from build123d import *

# Parameters (mm, degrees)
SKETCH1_W       = 22
SKETCH1_H       = 22
EXTRUDE1_DEPTH  = 7
SKETCH2_W       = 7
SKETCH2_H       = 7
EXTRUDE2_DEPTH  = 7
SKETCH3_W       = 7
SKETCH3_H       = 4
SKETCH3_W_2     = 4
SKETCH3_H_2     = 7
EXTRUDE3_DEPTH  = 7
SKETCH4_W       = 4
SKETCH4_H       = 4
EXTRUDE5_DEPTH  = 7
SKETCH5_R       = 2.55
EXTRUDE6_DEPTH  = 10
SKETCH6_R       = 1.025
EXTRUDE7_DEPTH  = 10
SKETCH7_R       = 1.025
EXTRUDE8_DEPTH  = 10
SKETCH8_R       = 1.025
EXTRUDE9_DEPTH  = 10
SKETCH9_R       = 1.025
EXTRUDE10_DEPTH = 10


with BuildPart() as part:
    # Sketch1 → Extrude1 (new body)
    with BuildSketch(Plane.XY):
        Rectangle(SKETCH1_W, SKETCH1_H)
    extrude(amount=EXTRUDE1_DEPTH)

    # Sketch2 → Extrude2 (cut)
    with BuildSketch(Plane.XY.offset(7)):
        with Locations((7.5, 7.5)):
            Rectangle(SKETCH2_W, SKETCH2_H)
        with Locations((-7.5, 7.5)):
            Rectangle(SKETCH2_W, SKETCH2_H)
        with Locations((-7.5, -7.5)):
            Rectangle(SKETCH2_W, SKETCH2_H)
        with Locations((7.5, -7.5)):
            Rectangle(SKETCH2_W, SKETCH2_H)
    extrude(amount=-EXTRUDE2_DEPTH, mode=Mode.SUBTRACT)

    # Sketch3 → Extrude3 (cut)
    with BuildSketch(Plane.XY.offset(7)):
        with Locations((-7.5, 0)):
            Rectangle(SKETCH3_W, SKETCH3_H)
        with Locations((0, 7.5)):
            Rectangle(SKETCH3_W_2, SKETCH3_H_2)
        with Locations((7.5, 0)):
            Rectangle(SKETCH3_W, SKETCH3_H)
        with Locations((0, -7.5)):
            Rectangle(SKETCH3_W_2, SKETCH3_H_2)
        Rectangle(SKETCH3_W_2, SKETCH3_H)
    extrude(amount=-EXTRUDE3_DEPTH, mode=Mode.SUBTRACT)

    # Sketch4 → Extrude5 (add)
    with BuildSketch(Plane.XY.offset(7)):
        Rectangle(SKETCH4_W, SKETCH4_H)
    extrude(amount=-EXTRUDE5_DEPTH)

    # Sketch5 → Extrude6 (cut)
    with BuildSketch(Plane.XY.offset(7)):
        Circle(SKETCH5_R)
    extrude(amount=-EXTRUDE6_DEPTH, mode=Mode.SUBTRACT)

    # Sketch6 → Extrude7 (cut)
    with BuildSketch(Plane(origin=(4, 0, 0), x_dir=(0, 0, -1), z_dir=(1, 0, 0))):
        with Locations((-3.14721043, 9.031360998)):
            Circle(SKETCH6_R)
    extrude(amount=-EXTRUDE7_DEPTH, mode=Mode.SUBTRACT)

    # Sketch7 → Extrude8 (cut)
    with BuildSketch(Plane.XZ.offset(4)):
        with Locations((-9, 3.526976634)):
            Circle(SKETCH7_R)
    extrude(amount=-EXTRUDE8_DEPTH, mode=Mode.SUBTRACT)

    # Sketch8 → Extrude9 (cut)
    with BuildSketch(Plane(origin=(4, 0, 0), x_dir=(0, 0, -1), z_dir=(1, 0, 0))):
        with Locations((-3.332535344, -9)):
            Circle(SKETCH8_R)
    extrude(amount=-EXTRUDE9_DEPTH, mode=Mode.SUBTRACT)

    # Sketch9 → Extrude10 (cut)
    with BuildSketch(Plane(origin=(0, 4, 0), x_dir=(1, 0, 0), z_dir=(0, 1, 0))):
        with Locations((9, -3.510451641)):
            Circle(SKETCH9_R)
    extrude(amount=-EXTRUDE10_DEPTH, mode=Mode.SUBTRACT)


solid = part.part
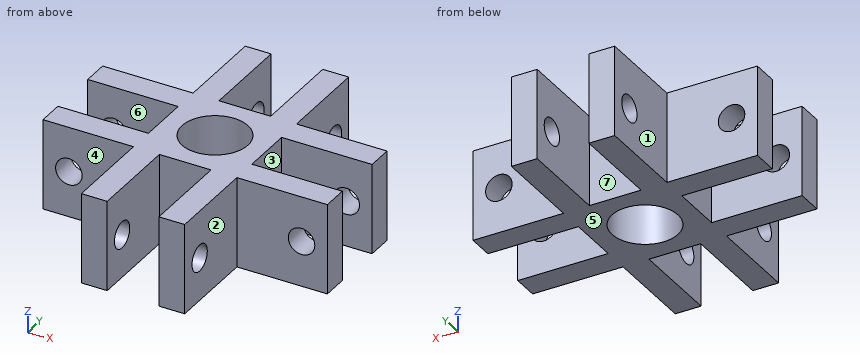
Verification items for the finished model (mm, model axes). Face numbers are marked on the shaded views. A direction names the side the tool comes from. Coordinates: 2 decimals unless noted, no trailing zeros. Write each loop counter-clockwise with the first axis right and the second up, starting at its lowest first coordinate (ties: lowest second). Pieces come first, ordered by that corner, then holes. Notation, with made-up numbers: M 11.5,59.5 L 56.5,59.5 A30 ccw 56.5,89.5 Z; hole C 80.25,29 d8. An arc over 180 degrees is marked long. One line per question, with ' | ' between items.
1) Sectioned sample at D-D on y = 0. Record the cut outline in (x, z).
Solutions:
outline: M -4,0 L -2.55,0 L -2.55,7 L -4,7 Z; M 2.55,0 L 4,0 L 4,7 L 2.55,7 Z
2) Sectioned sample at A-A on x = -7. Record the cut outline in (y, z), then the cut area to 3 significant figures.
Solutions:
outline: M -4,0 L -2,0 L -2,7 L -4,7 Z; M 2,0 L 4,0 L 4,7 L 2,7 Z | area: 28.0 mm^2
3) Material ranges on L1, parallel to Y at x = 5, z = 3; L2, parallel to Z at x = -9, y = -2.45, recorded low to high.
Solutions:
L1: -4 to -2, 2 to 4 | L2: 0 to 2.5, 4.55 to 7
4) Access from +Z, -Z, +X, -X, +Y, -Y to the whole of each face (thin tool, end or side, straight path). Record for the marked faces 1, 2, 3 and 4.
Solutions:
face 1: +Z, -Z, -X, +Y | face 2: +Z, -Z, +X, -Y | face 3: +Z, -Z, +X | face 4: +Z, -Z, -X, -Y
5) Sectioned sample at B-B on y = -9. Record the cut outline in (x, z), then the cut area to 3 significant figures.
Solutions:
outline: M -4,0 L -2,0 L -2,2.31 L -4,2.31 Z; M -4,4.36 L -2,4.36 L -2,7 L -4,7 Z; M 2,0 L 4,0 L 4,2.31 L 2,2.31 Z; M 2,4.36 L 4,4.36 L 4,7 L 2,7 Z | area: 19.8 mm^2
6) Depth check by flat-ended pin: pin 1 Ø2.5 at (x, z) = (9, 3.51) entering from -Y; pin 2 Ø2 at (y, z) = (-8, 4) entering from +X; pin 3 Ø2 at (y, z) = (6.5, 3.5) entering from -X. Enter the tip coordinate at first touch or a pass-through.
Solutions:
pin 1: y = -4 | pin 2: x = 4 | pin 3: x = -4
7) Release check for a two-part mould opening along Y. For the marked faces 5, 6 and 7 record: +Y half, -Y half, draft (parallel to the pull), parting line (faces both ways), or undercut.
Solutions:
face 5: draft | face 6: undercut | face 7: +Y half
